Geometry: final body of the model. Coordinates: model frame, mm. A direction names the side the tool comes from. Give positions to 0.01 mm unless a question says otherwise; leave off trailing zeros. Order: outer loops, then holes, each group sorted by start corner. A loop starts at its lowest first (then second) coordinate and runs counter-clockwise, first axis right, second up. Notation, with made-up numbers: (-17, 73.25) - (31, 73.25) arc R32 ccw to (31, 110.25) - close; hole circle Ø10 at (-37.75, -31.75). An arc over 180 degrees is marked (long way). One line per item, written item: value.
```python
from build123d import *

# Parameters (mm, degrees)
ESQUISSE1_W                               = 40
ESQUISSE1_H                               = 30
BOSS_EXTRU_1_DEPTH                        = 5
BOSS_EXTRU_2_DEPTH                        = 5
TROUS_DE_CENTRAGE_1_0MM1_D                = 22
D_GAGEMENT_M34_D                          = 3.6
TROU_POUR_TARAUDAGE_POUR_TROU_TARAUD_M2_D = 1.6


with BuildPart() as part:
    # Esquisse1 → Boss.-Extru.1 (new body)
    with BuildSketch(Plane.XY):
        with Locations((-1, -4.421052632)):
            Rectangle(ESQUISSE1_W, ESQUISSE1_H)
    extrude(amount=BOSS_EXTRU_1_DEPTH)

    # Esquisse2 → Boss.-Extru.2 (add)
    with BuildSketch(Plane.XY.offset(5)):
        with BuildLine():
            Line((-13.5, 10.578947368), (11.5, 10.578947368))
            Line((11.5, 10.578947368), (11.5, 23.078947368))
            ThreePointArc((11.5, 23.078947368), (-1, 35.578947368), (-13.5, 23.078947368))
            Line((-13.5, 23.078947368), (-13.5, 10.578947368))
        make_face()
    extrude(amount=-BOSS_EXTRU_2_DEPTH)

    # Trous de centrage Ø1.0mm1 (through all)
    with Locations(Plane.XY.offset(5)):
        with Locations((-1, 23.078947368)):
            Hole(TROUS_DE_CENTRAGE_1_0MM1_D / 2)

    # Dégagement M34 (through all)
    with Locations(Plane.XY.offset(5)):
        with Locations((9, 7.578947368), (-11, 7.578947368), (-11, -12.421052632), (9, -12.421052632)):
            Hole(D_GAGEMENT_M34_D / 2)

    # Trou pour taraudage pour trou taraudé M23 (through all)
    with Locations(Plane(origin=(11.5, 0, 0), x_dir=(0, 0, -1), z_dir=(1, 0, 0))):
        with Locations((-2.5, 23.078947368)):
            Hole(TROU_POUR_TARAUDAGE_POUR_TROU_TARAUD_M2_D / 2)


solid = part.part
```
1) First-contact query: pin 1 (6 mm diameter, centred on x = -11, y = -12.42, fed in from -Z). Flat tip, straight axial feed; report the tip coordinate or a pass-through.
Answers below:
pin 1: z = 0
2) Section C-C, the plane y = 14. Return loops of the section in (x, z), then the cut area to 3 significant figures.
Answers below:
outline: (-13.5, 0) - (-7.21, 0) - (-7.21, 5) - (-13.5, 5) - close; (5.21, 0) - (11.5, 0) - (11.5, 5) - (5.21, 5) - close
area: 62.9 mm^2
3) Section B-B, the plane z = 2.5. Return loops of the section in (x, y).
Answers below:
outline: (-21, -19.42) - (19, -19.42) - (19, 10.58) - (11.5, 10.58) - (11.5, 22.28) - (9.97, 22.28) arc R11 cw to (-11.97, 22.28) - (-13.5, 22.28) - (-13.5, 10.58) - (-21, 10.58) - close; (-13.47, 23.88) - (-11.97, 23.88) arc R11 cw to (9.97, 23.88) - (11.47, 23.88) arc R12.5 ccw to start; hole circle Ø3.6 at (-11, -12.42); hole circle Ø3.6 at (-11, 7.58); hole circle Ø3.6 at (9, -12.42); hole circle Ø3.6 at (9, 7.58)
4) Section D-D, the plane x = 8.5. Return loops of the section in (y, z), then the cut area to 3 significant figures.
Answers below:
outline: (-19.42, 0) - (-14.15, 0) - (-14.15, 5) - (-19.42, 5) - close; (-10.69, 0) - (5.85, 0) - (5.85, 5) - (-10.69, 5) - close; (9.31, 0) - (17.53, 0) - (17.53, 5) - (9.31, 5) - close; (28.62, 0) - (31.2, 0) - (31.2, 5) - (28.62, 5) - close
area: 163 mm^2
5) Mould query, pull axis Z, two halves, no side actions, for faces 4 (the face through (-1, -4, 5)), 5 (the face through (10.725, 23.754, 2.93)), 6 (the face through (-21, -5, 2)). Classes: released by +Z, released by -Z, zero draft, split by the parting line, or undercut.
Answers below:
face 4: released by +Z
face 5: undercut
face 6: zero draft
6) Set-up query: faces 1 (the face through (-11.161, 18.866, 2.465)), 2 (the face through (11.5, 17, 3)), 3 (the face through (-17, 10.579, 2)). Return all of +Z, -Z, +X, -X, +Y, -Y with unobstructed straight access to the full face (end or side cutting, diameter ignored); none if empty.
Answers below:
face 1: +Z, -Z
face 2: +Z, -Z, +X, +Y
face 3: +Z, -Z, -X, +Y
7) Material intervals for line 1 along X through (y, z) = (23, 1.35); line 2 along Y through (x, z) = (-10, 0.5); line 3 along Y through (x, z) = (9, 3.9), sorted ascending.
Answers below:
line 1: -13.5 to -12, 10 to 11.5
line 2: -19.42 to -13.92, -10.92 to 6.08, 9.08 to 16.75, 29.4 to 31.75
line 3: -19.42 to -14.22, -10.62 to 5.78, 9.38 to 18.5, 27.66 to 30.58
8) Section A-A, the plane x = -1. Return loops of the section in (y, z), then the cut area to 3 significant figures.
Answers below:
outline: (-19.42, 0) - (12.08, 0) - (12.08, 5) - (-19.42, 5) - close; (34.08, 0) - (35.58, 0) - (35.58, 5) - (34.08, 5) - close
area: 165 mm^2
